```python
from build123d import *

# Parameters (mm, degrees)
SKETCH_1_W          = 55.5
SKETCH_1_H          = 23.5
EXTRUDE_1_DEPTH     = 1.2
FILLET_1_R          = 2
SKETCH_2_W          = 53.7
SKETCH_2_H          = 22.3
EXTRUDE_2_DEPTH     = 0.6
SKETCH_3_W          = 15
SKETCH_3_H          = 13.5
SKETCH_3_W_2        = 14
SKETCH_3_H_2        = 14
CUT_EXTRUDE_1_DEPTH = 3
FILLET_2_R          = 1
SKETCH_4_W          = 15.5
SKETCH_4_H          = 3.997435945
CUT_EXTRUDE_2_DEPTH = 0.5
SKETCH_5_W          = 53.5
SKETCH_5_H          = 1.5
EXTRUDE_3_DEPTH     = 6.5
FILLET_3_R          = 1
SKETCH_6_W          = 1.5
SKETCH_6_H          = 4
EXTRUDE_4_DEPTH     = 3.75
CHAMFER_1_SIZE      = 2
FILLET_4_R          = 1.5


with BuildPart() as part:
    # 草图1 → 凸台-拉伸1 (new body)
    with BuildSketch(Plane(origin=(0, 0, 0), x_dir=(1, 0, 0), z_dir=(0, 1, 0))):
        Rectangle(SKETCH_1_W, SKETCH_1_H)
    extrude(amount=EXTRUDE_1_DEPTH)

    # 圆角1
    fillet_1_edges = [part.edges().sort_by_distance(p)[0] for p in [
        (27.75, 0.6, 11.75),
        (-27.75, 0.6, 11.75),
        (-27.75, 0.6, -11.75),
        (27.75, 0.6, -11.75),
    ]]
    fillet(fillet_1_edges, radius=FILLET_1_R)

    # 草图2 → 凸台-拉伸2 (add)
    with BuildSketch(Plane.XZ):
        Rectangle(SKETCH_2_W, SKETCH_2_H)
    extrude(amount=EXTRUDE_2_DEPTH)

    # 草图3 → 切除-拉伸1 (cut)
    with BuildSketch(Plane.XZ.offset(0.6)):
        with Locations((-17.65, 3)):
            Rectangle(SKETCH_3_W, SKETCH_3_H)
        with Locations((1.05, 3.85)):
            Rectangle(SKETCH_3_W_2, SKETCH_3_H_2)
        with Locations((18.75, 3.85)):
            Rectangle(SKETCH_3_W_2, SKETCH_3_H_2)
    extrude(amount=-CUT_EXTRUDE_1_DEPTH, mode=Mode.SUBTRACT)

    # 圆角2
    fillet_2_edges = [part.edges().sort_by_distance(p)[0] for p in [
        (-25.15, 0.3, -3.75),
        (-25.15, 0.3, 9.75),
        (-10.15, 0.3, 9.75),
        (-10.15, 0.3, -3.75),
        (-5.95, 0.3, -3.15),
        (-5.95, 0.3, 10.85),
        (8.05, 0.3, 10.85),
        (8.05, 0.3, -3.15),
        (11.75, 0.3, -3.15),
        (11.75, 0.3, 10.85),
        (25.75, 0.3, 10.85),
        (25.75, 0.3, -3.15),
    ]]
    fillet(fillet_2_edges, radius=FILLET_2_R)

    # 草图4 → 切除-拉伸2 (cut)
    with BuildSketch(Plane(origin=(0, 1.2, 0), x_dir=(1, 0, 0), z_dir=(0, 1, 0))):
        with Locations((-20, -3.751282028)):
            Rectangle(SKETCH_4_W, SKETCH_4_H)
    extrude(amount=-CUT_EXTRUDE_2_DEPTH, mode=Mode.SUBTRACT)

    # 草图5 → 凸台-拉伸3 (add)
    with BuildSketch(Plane(origin=(0, 1.2, 0), x_dir=(1, 0, 0), z_dir=(0, 1, 0))):
        with Locations((0, 6.804632487)):
            Rectangle(SKETCH_5_W, SKETCH_5_H)
    extrude(amount=EXTRUDE_3_DEPTH)

    # 圆角3
    fillet_3_edges = [part.edges().sort_by_distance(p)[0] for p in [
        (26.75, 7.7, -6.804632487),
        (-26.75, 7.7, -6.804632487),
    ]]
    fillet(fillet_3_edges, radius=FILLET_3_R)

    # 草图6 → 凸台-拉伸4 (add)
    with BuildSketch(Plane(origin=(0, 1.2, 0), x_dir=(1, 0, 0), z_dir=(0, 1, 0))):
        with Locations((9, 4.054632487)):
            Rectangle(SKETCH_6_W, SKETCH_6_H)
        with Locations((-11, 4.054632487)):
            Rectangle(SKETCH_6_W, SKETCH_6_H)
    extrude(amount=EXTRUDE_4_DEPTH)

    # 倒角1
    chamfer_1_edges = [part.edges().sort_by_distance(p)[0] for p in [
        (9, 4.95, -2.054632487),
        (-11, 4.95, -2.054632487),
    ]]
    chamfer(chamfer_1_edges, length=CHAMFER_1_SIZE)

    # 圆角4
    fillet_4_edges = [part.edges().sort_by_distance(p)[0] for p in [
        (-26.85, -0.3, 11.15),
        (-26.85, -0.3, -11.15),
        (26.85, -0.3, -11.15),
        (26.85, -0.3, 11.15),
    ]]
    fillet(fillet_4_edges, radius=FILLET_4_R)


solid = part.part
```
For this review, take the finished solid that the model builds, in its own axes (mm). A direction names the side the tool comes from. Give positions to 0.01 mm unless a question says otherwise; leave off trailing zeros. Write each loop counter-clockwise with the first axis right and the second up, starting at its lowest first coordinate (ties: lowest second). Pieces come first, ordered by that corner, then holes. Notation, with made-up numbers: M 13,-26.75 L 26,-26.75 A24 ccw 26,-11.75 Z; hole C -31,56 d11. An arc over 180 degrees is marked long. Answer as a JSON object with one key per item and string values. Group by question number.
Item 1: Consider section B-B on x = 19.5. Write out the cut boundary in (y, z), plus the area to 3 significant figures.
Item 2: Draft analysis for pull direction Z (two halves, no side actions). For faces 1 (the cylindrical face through (26.4, -0.3, 10.72)), 2 (the cylindrical face through (-24.849, 0.313, -3.465)), 3 (the cylindrical face through (12.051, 0.313, 10.565)), 4 (the cylindrical face through (26.465, 7.399, -6.815)), state which applies: +Z half, -Z half, draft (parallel to the pull), parting line (faces both ways), or undercut.
Item 3: For pin 1 Ø3 at (x, z) = (10, 4) entering from +Y; pin 2 Ø1 at (x, y) = (11.5, 2.5) entering from -Z; pin 3 Ø0.7 at (x, y) = (-2, -0.5) entering from -Z, all flat-tipped, find the tip position at first contact; note any pin that passes through.
Item 4: Tool access review of faces 5 (the cylindrical face through (27.18, 0.61, -11.15)), 6 (the flat face through (-25.15, 0, 3)), 7 (the flat face through (-11, 4.95, -5)), 8 (the cylindrical face through (-26.42, -0.3, 10.7)): name each direction out of +Z, -Z, +X, -X, +Y, -Y from which nothing blocks a thin tool from reaching the whole face with its end or side.
Item 5: For probe 1 along X at (y, z) = (0.5, 5.25); probe 2 along Z at (x, y) = (-21, 2.75); probe 3 along Y at (x, z) = (13, -4.25), list the stretches that pass through material, from the lowest coordinate up. Write a range as [from, to].
Item 6: Consider section A-A on z = 6.25. Write out the cut boundary in (x, y), plus the area to 3 significant figures.
Item 7: Consider section C-C on y = 1.75. Write out the cut boundary in (x, z), plus the area to 4 significant figures.
Item 8: Consider section D-D on z = -8.75. Write out the cut boundary in (x, y).
Check result:
{
 "1": {"outline": "M -0.6,-11.15 L 0,-11.15 L 0,-11.75 L 1.2,-11.75 L 1.2,-7.55 L 7.7,-7.55 L 7.7,-6.05 L 1.2,-6.05 L 1.2,-3.15 L -0.6,-3.15 Z; M -0.6,10.85 L 1.2,10.85 L 1.2,11.75 L 0,11.75 L 0,11.15 L -0.6,11.15 Z", "area": "26.1 mm^2"},
 "2": {"face 1": "+Z half", "face 2": "undercut", "face 3": "undercut", "face 4": "draft"},
 "3": {"pin 1": "stops at y = 1.2", "pin 2": "stops at z = -7.55", "pin 3": "stops at z = -11.15"},
 "4": {"face 5": "-Z, +X, +Y, -Y", "face 6": "+Y, -Y", "face 7": "+Z, +X, -X, +Y", "face 8": "+Z, -X, -Y"},
 "5": {"probe 1": "x = [-27.75, -25.15], [-10.15, -5.95], [8.05, 11.75], [25.75, 27.75]", "probe 2": "z = [-7.55, -6.05]", "probe 3": "y = [-0.6, 1.2]"},
 "6": {"outline": "M -27.75,0 L -26.85,0 L -26.85,-0.6 L -25.15,-0.6 L -25.15,1.2 L -27.75,1.2 Z; M -10.15,-0.6 L -5.95,-0.6 L -5.95,1.2 L -10.15,1.2 Z; M 8.05,-0.6 L 11.75,-0.6 L 11.75,1.2 L 8.05,1.2 Z; M 25.75,-0.6 L 26.85,-0.6 L 26.85,0 L 27.75,0 L 27.75,1.2 L 25.75,1.2 Z", "area": "21.4 mm^2"},
 "7": {"outline": "M -26.75,-7.55 L 26.75,-7.55 L 26.75,-6.05 L 9.75,-6.05 L 9.75,-2.05 L 8.25,-2.05 L 8.25,-6.05 L -10.25,-6.05 L -10.25,-2.05 L -11.75,-2.05 L -11.75,-6.05 L -26.75,-6.05 Z", "area": "92.25 mm^2"},
 "8": {"outline": "M -27.75,0 L -26.85,0 L -26.85,-0.6 L 26.85,-0.6 L 26.85,0 L 27.75,0 L 27.75,1.2 L -27.75,1.2 Z"}
}
